```python
from build123d import *

# Parameters (mm, degrees)
F0_R     = 1.524
F1_DEPTH = 2.54


# Not quite as in the source:
# - a feature names something its author has since deleted; it is built from what else it names


with BuildPart() as f1:
    # F0 (on Top) → F1 (new body)
    with BuildSketch(Plane.XY):
        with BuildLine():
            Line((-19.0341994166, 42.3401940286), (-6.35, 31.75))
            Line((-6.35, 31.75), (-6.35, -19.05))
            ThreePointArc((-6.35, -19.05), (-4.4901280605, -23.5401280605), (0, -25.4))
            ThreePointArc((0, -25.4), (4.4901280605, -23.5401280605), (6.35, -19.05))
            Line((6.35, -19.05), (6.35, 36.83))
            Line((6.35, 36.83), (-6.35, 47.4333861299))
            Line((-6.35, 47.4333861299), (-6.35, 57.15))
            Line((-6.35, 57.15), (-6.35, 63.5))
            Line((-6.35, 63.5), (-19.0341994166, 63.5))
            Line((-19.0341994166, 63.5), (-19.0341994166, 42.3401940286))
        make_face()
        with Locations((0, -19.05)):
            Circle(F0_R, mode=Mode.SUBTRACT)
        with Locations((0, 16.51)):
            Circle(F0_R, mode=Mode.SUBTRACT)
    extrude(amount=F1_DEPTH)


solid = f1.part
```
Input: part model. Units: mm. Frame: model coordinates. Coordinates: 2 decimals unless noted, no trailing zeros. Write each loop counter-clockwise with the first axis right and the second up, starting at its lowest first coordinate (ties: lowest second). Pieces come first, ordered by that corner, then holes.
1) Section B-B on y = -7.5. Output: boundary loops of the cut face in (x, z), and give its area (3 significant figures).
2) Mould query, pull axis X, two halves, no side actions, for faces 1 (the flat face through (-6.35, 7, 1)), 2 (the cylindrical face through (-0.2, 18.02, 1.25)), 3 (the flat face through (-6.35, 55, 1)), 4 (the flat face through (-4, 20, 2.54)). Classes: pulls with the +X half, pulls with the -X half, needs draft (parallel to the pull), parting line crosses it, or undercut.
3) Section A-A on y = 16.51. Output: boundary loops of the cut face in (x, z), and give its area (3 significant figures).
4) Material intervals for line 1 along Y through (x, z) = (0.75, 1.4); line 2 along X through (y, z) = (56, 0.6); line 3 along Y through (x, z) = (-2, 1.1), sorted ascending.
5) Pin query (flat end, axial travel): pin 1 Ø8 at (x, y) = (-12, 38.5) entering from -Z; pin 2 Ø1 at (x, z) = (-4.5, 2) entering from -Y; pin 3 Ø1.3 at (y, z) = (51.5, 2) entering from +X; pin 4 Ø1.8 at (x, y) = (0, 16.51) entering from -Z. Return the tip coordinate at first contact, or that it passes through.
6) Section C-C on x = -9. Output: boundary loops of the cut face in (y, z), and give its area (3 significant figures).
Check result:
1. outline: (-6.35, 0) - (6.35, 0) - (6.35, 2.54) - (-6.35, 2.54) - close
1. area: 32.3 mm2
2. face 1: pulls with the -X half
2. face 2: undercut
2. face 3: pulls with the +X half
2. face 4: needs draft
3. outline: (-6.35, 0) - (-1.52, 0) - (-1.52, 2.54) - (-6.35, 2.54) - close; (1.52, 0) - (6.35, 0) - (6.35, 2.54) - (1.52, 2.54) - close
3. area: 24.5 mm2
4. line 1: y = -25.36 to -20.38, -17.72 to 15.18, 17.84 to 41.51
4. line 2: x = -19.03 to -6.35
4. line 3: y = -25.08 to 43.8
5. pin 1: stops at z = 0
5. pin 2: stops at y = -23.98
5. pin 3: stops at x = -6.35
5. pin 4: passes through
6. outline: (33.96, 0) - (63.5, 0) - (63.5, 2.54) - (33.96, 2.54) - close
6. area: 75.0 mm2
